Part model, mm, in its own coordinate system. A direction names the side the tool comes from. Round coordinates to 2 decimals unless told otherwise and drop trailing zeros. Write each loop counter-clockwise with the first axis right and the second up, starting at its lowest first coordinate (ties: lowest second). Pieces come first, ordered by that corner, then holes. Notation, with made-up numbers: M -27.75,31.25 L 0.25,31.25 A29 cw 0.25,60.25 Z; hole C 57,41 d8. An arc over 180 degrees is marked long. Use a Markdown table: item, result. Add a question column.
1) Slice it at C-C on z = 12.5. Write the cut outline in (x, y), plus the area to 3 significant figures.
2) Which spindle directions (+Z, -Z, +X, -X, +Y, -Y) get a long thin tool onto all of the face, cutting with end or side? Do faces 1 (the face through (18, -1, 27)), 2 (the face through (20, -33, 44)), 3 (the face through (-21, -33, 43)). Say none if no direction does.
3) Slice it at B-B on x = 3. Write the cut outline in (y, z).
4) Slice it at D-D on y = 15. Write the cut outline in (x, z).
5) Drop flat-ended pins along their axis: P1, Ø2, axis at x = 20, z = 46, coming from the +Y side; P2, Ø4.5, axis at x = -20, z = 45, coming from the +Y side; P3, Ø1.2, axis at x = 21, z = 44.5, coming from the +Y side; P4, Ø4.5, axis at x = -19, z = 45.5, coming from the +Y side. Give the stop position or say it passes through.
6) Slice it at A-A on y = 34. Write the cut outline in (x, z), plus the area to 3 significant figures.
7) Two-plate mould, pull along Y, no slides. Class faces 4 (the face through (20, 38, 47)), 5 (the face through (-22, -1, 28)), 6 (the face through (0, 57, -2)): released by +Y, released by -Y, zero draft, split by the parting line, or undercut.
8) Wall check: probe 1 along X at (y, z) = (-26, 3); probe 2 along Y at (x, z) = (-2.5, 30); probe 3 along Z at (x, y) = (6.5, 42.5). Give the ranges that are in metal, low to high.
```python
from build123d import *

# Parameters (mm, degrees)
F0_W         = 36
F0_H         = 108
F1_DEPTH     = 55
F2_T         = 4
F3_T1_DEPTH  = 66.5
F3_T3_DEPTH  = 34
F3_T5_DEPTH  = 106
F3_S9_W      = 5
F3_S9_H      = 5
F3_T10_DEPTH = 5
F3_S15_W     = 5
F3_S15_H     = 5
F3_T16_DEPTH = 5
F3_S21_W     = 5
F3_S21_H     = 5
F3_T22_DEPTH = 5
F3_S27_W     = 5
F3_S27_H     = 5
F3_T28_DEPTH = 5
F4_W         = 10
F4_H         = 5
F5_DEPTH     = 44.001
F6_SIZE      = 3


# Not quite as in the source:
# - a fillet or chamfer that OpenCascade refuses, or shapes differently, is made with other operations: its cross-section is extruded or revolved along the edge and cut away or added


with BuildPart() as f1:
    # F0 (on Top) → F1 (new body)
    with BuildSketch(Plane.XY):
        Rectangle(F0_W, F0_H)
    extrude(amount=F1_DEPTH)

    # F2
    f2_openings = [f1.faces().sort_by_distance(p)[0] for p in [
        (0, 0, 55),
    ]]
    offset(amount=F2_T, openings=f2_openings, kind=Kind.INTERSECTION)

    # F3: fillet of radius 5 on 8 edges, made by hand

    # F3_s2 → F3_t1 (cut)
    with BuildSketch(Plane.XY.offset(1)):
        with BuildLine():
            ThreePointArc((-17, -58), (-20.5355339059, -56.5355339059), (-22, -53))
            Line((-22, -53), (-22, -58))
            Line((-22, -58), (-17, -58))
        make_face()
        with BuildLine():
            ThreePointArc((17, -58), (20.5355339059, -56.5355339059), (22, -53))
            Line((22, -53), (22, -58))
            Line((22, -58), (17, -58))
        make_face()
        with BuildLine():
            ThreePointArc((22, 53), (20.5355339059, 56.5355339059), (17, 58))
            Line((17, 58), (22, 58))
            Line((22, 58), (22, 53))
        make_face()
        with BuildLine():
            ThreePointArc((-17, 58), (-20.5355339059, 56.5355339059), (-22, 53))
            Line((-22, 53), (-22, 58))
            Line((-22, 58), (-17, 58))
        make_face()
    extrude(amount=F3_T1_DEPTH, mode=Mode.SUBTRACT)

    # F3_s4 → F3_t3 (cut)
    with BuildSketch(Plane.YZ.offset(-17)):
        with BuildLine():
            ThreePointArc((-58, 1), (-56.5355339059, -2.5355339059), (-53, -4))
            Line((-53, -4), (-58, -4))
            Line((-58, -4), (-58, 1))
        make_face()
        with BuildLine():
            ThreePointArc((58, 1), (56.5355339059, -2.5355339059), (53, -4))
            Line((53, -4), (58, -4))
            Line((58, -4), (58, 1))
        make_face()
    extrude(amount=F3_T3_DEPTH, mode=Mode.SUBTRACT)

    # F3_s6 → F3_t5 (cut)
    with BuildSketch(Plane.XZ.offset(-53)):
        with BuildLine():
            ThreePointArc((22, 1), (20.5355339059, -2.5355339059), (17, -4))
            Line((17, -4), (22, -4))
            Line((22, -4), (22, 1))
        make_face()
        with BuildLine():
            ThreePointArc((-22, 1), (-20.5355339059, -2.5355339059), (-17, -4))
            Line((-17, -4), (-22, -4))
            Line((-22, -4), (-22, 1))
        make_face()
    extrude(amount=F3_T5_DEPTH, mode=Mode.SUBTRACT)


with BuildPart() as f3_tool8:
    # F3_s9 → F3_t10 (new body)
    with BuildSketch(Plane.YZ.offset(-17)):
        with Locations((-55.5, -1.5)):
            Rectangle(F3_S9_W, F3_S9_H)
    extrude(amount=-F3_T10_DEPTH)

    # F3_s11 → F3_t12 (revolve, cut)
    with BuildSketch(Plane(origin=(-17, -53, 1), x_dir=(0, 0.7071067812, 0.7071067812), z_dir=(0, -0.7071067812, 0.7071067812))):
        with BuildLine():
            ThreePointArc((0, -5), (5, 0), (0, 5))
            Line((0, 5), (0, -5))
        make_face()
    revolve(axis=Axis((-17, -53, 1), (-1, 0, 0)), mode=Mode.SUBTRACT)


with BuildPart() as f1_1:
    add(f1.part)

    # F3_t7: cut F3_tool8
    add(f3_tool8.part, mode=Mode.SUBTRACT)


with BuildPart() as f3_tool14:
    # F3_s15 → F3_t16 (new body)
    with BuildSketch(Plane.XY.offset(1)):
        with Locations((19.5, -55.5)):
            Rectangle(F3_S15_W, F3_S15_H)
    extrude(amount=-F3_T16_DEPTH)

    # F3_s17 → F3_t18 (revolve, cut)
    with BuildSketch(Plane(origin=(17, -53, 1), x_dir=(-0.7071067812, 0.7071067812, 0), z_dir=(-0.7071067812, -0.7071067812, 0))):
        with BuildLine():
            ThreePointArc((0, -5), (5, 0), (0, 5))
            Line((0, 5), (0, -5))
        make_face()
    revolve(axis=Axis((17, -53, 1), (0, 0, -1)), mode=Mode.SUBTRACT)


with BuildPart() as f1_2:
    add(f1_1.part)

    # F3_t13: cut F3_tool14
    add(f3_tool14.part, mode=Mode.SUBTRACT)


with BuildPart() as f3_tool20:
    # F3_s21 → F3_t22 (new body)
    with BuildSketch(Plane.XZ.offset(-53)):
        with Locations((19.5, -1.5)):
            Rectangle(F3_S21_W, F3_S21_H)
    extrude(amount=-F3_T22_DEPTH)

    # F3_s23 → F3_t24 (revolve, cut)
    with BuildSketch(Plane(origin=(17, 53, 1), x_dir=(-0.7071067812, 0, 0.7071067812), z_dir=(-0.7071067812, 0, -0.7071067812))):
        with BuildLine():
            ThreePointArc((0, -5), (5, 0), (0, 5))
            Line((0, 5), (0, -5))
        make_face()
    revolve(axis=Axis((17, 53, 1), (0, 1, 0)), mode=Mode.SUBTRACT)


with BuildPart() as f1_3:
    add(f1_2.part)

    # F3_t19: cut F3_tool20
    add(f3_tool20.part, mode=Mode.SUBTRACT)


with BuildPart() as f3_tool26:
    # F3_s27 → F3_t28 (new body)
    with BuildSketch(Plane.XZ.offset(-53)):
        with Locations((-19.5, -1.5)):
            Rectangle(F3_S27_W, F3_S27_H)
    extrude(amount=-F3_T28_DEPTH)

    # F3_s29 → F3_t30 (revolve, cut)
    with BuildSketch(Plane(origin=(-17, 53, 1), x_dir=(0.7071067812, 0, 0.7071067812), z_dir=(-0.7071067812, 0, 0.7071067812))):
        with BuildLine():
            ThreePointArc((0, -5), (5, 0), (0, 5))
            Line((0, 5), (0, -5))
        make_face()
    revolve(axis=Axis((-17, 53, 1), (0, 1, 0)), mode=Mode.SUBTRACT)


with BuildPart() as f1_4:
    add(f1_3.part)

    # F3_t25: cut F3_tool26
    add(f3_tool26.part, mode=Mode.SUBTRACT)

    # F4 (on face) → F5 (cut, through all)
    with BuildSketch(Plane(origin=(-22, 0, 0), x_dir=(0, -1, 0), z_dir=(-1, 0, 0))):
        with Locations((-33, 47.5)):
            Rectangle(F4_W, F4_H)
        with Locations((33, 47.5)):
            Rectangle(F4_W, F4_H)
    extrude(amount=-F5_DEPTH, mode=Mode.SUBTRACT)

    # F6
    f6_edges = [f1_4.edges().sort_by_distance(p)[0] for p in [
        (-22, 33, 45),
        (-22, -33, 45),
        (22, -33, 45),
        (22, 33, 45),
    ]]
    chamfer(f6_edges, length=F6_SIZE)


solid = f1_4.part
```
Entries:
| question | item | result |
|---|---|---|
| 1 | outline | M -22,-53 A5 ccw -17,-58 L 17,-58 A5 ccw 22,-53 L 22,53 A5 ccw 17,58 L -17,58 A5 ccw -22,53 Z; hole M -18,-54 L 18,-54 L 18,54 L -18,54 Z |
| 1 | area | 1,190 mm^2 |
| 2 | face 1 | +Z |
| 2 | face 2 | +X |
| 2 | face 3 | -X |
| 3 | outline | M -58,1 A5 ccw -53,-4 L 53,-4 A5 ccw 58,1 L 58,55 L 54,55 L 54,0 L -54,0 L -54,55 L -58,55 Z |
| 4 | outline | M -22,1 A5 ccw -17,-4 L 17,-4 A5 ccw 22,1 L 22,55 L 18,55 L 18,0 L -18,0 L -18,55 L -22,55 Z |
| 5 | P1 | stops at y = 57.58 |
| 5 | P2 | stops at y = 57.94 |
| 5 | P3 | stops at y = 56.67 |
| 5 | P4 | stops at y = 58 |
| 6 | outline | M -22,1 A5 ccw -17,-4 L 17,-4 A5 ccw 22,1 L 22,42 L 19,45 L 18,45 L 18,0 L -18,0 L -18,45 L -19,45 L -22,42 Z; M -22,50 L -18,50 L -18,55 L -22,55 Z; M 18,50 L 22,50 L 22,55 L 18,55 Z |
| 6 | area | 556 mm^2 |
| 7 | face 4 | undercut |
| 7 | face 5 | zero draft |
| 7 | face 6 | released by +Y |
| 8 | probe 1 | x = -22 to -18, 18 to 22 |
| 8 | probe 2 | y = -58 to -54, 54 to 58 |
| 8 | probe 3 | z = -4 to 0 |
